from build123d import *

# Parameters (mm, degrees)
DODANIE_WYCI_GNI_CIE1_DEPTH = 20
SZKIC2_W                    = 20
SZKIC2_H                    = 40
DODANIE_WYCI_GNI_CIE2_DEPTH = 20
WYTNIJ_WYCI_GNI_CIE1_DEPTH  = 20
ZAOKR_GLENIE1_R             = 10
ZAOKR_GLENIE2_R             = 10


with BuildPart() as part:
    # Szkic1 → Dodanie-wyciągnięcie1 (new body)
    with BuildSketch(Plane.XY):
        with BuildLine():
            Line((0, 0), (40, 0))
            Line((40, 0), (40, 20))
            ThreePointArc((40, 20), (34.142135624, 34.142135624), (20, 40))
            Line((20, 40), (0, 40))
            Line((0, 40), (0, 0))
        make_face()
    extrude(amount=DODANIE_WYCI_GNI_CIE1_DEPTH)

    # Szkic2 → Dodanie-wyciągnięcie2 (add)
    with BuildSketch(Plane.XY.offset(20)):
        with Locations((10, 20)):
            Rectangle(SZKIC2_W, SZKIC2_H)
    extrude(amount=DODANIE_WYCI_GNI_CIE2_DEPTH)

    # Szkic3 → Wytnij-wyciągnięcie1 (cut)
    with BuildSketch(Plane(origin=(20, 0, 0), x_dir=(0, 0, -1), z_dir=(1, 0, 0))):
        Polygon((-40, 20), (-30, 20), (-20, 20), (-20, 40), (-40, 40), align=None)
    extrude(amount=-WYTNIJ_WYCI_GNI_CIE1_DEPTH, mode=Mode.SUBTRACT)

    # Zaokrąglenie1
    zaokr_glenie1_edges = [part.edges().sort_by_distance(p)[0] for p in [
        (10, 20, 20),
    ]]
    fillet(zaokr_glenie1_edges, radius=ZAOKR_GLENIE1_R)

    # Zaokrąglenie2
    zaokr_glenie2_edges = [part.edges().sort_by_distance(p)[0] for p in [
        (10, 20, 40),
    ]]
    fillet(zaokr_glenie2_edges, radius=ZAOKR_GLENIE2_R - 0.0001)  # a hair under: the kernel refuses the full size


solid = part.part
Read the model definition and answer for the solid it produces. Units are mm, in the model's axes. A direction names the side the tool comes from. Round coordinates to 2 decimals unless told otherwise and drop trailing zeros. Write each loop counter-clockwise with the first axis right and the second up, starting at its lowest first coordinate (ties: lowest second). Pieces come first, ordered by that corner, then holes. Notation, with made-up numbers: (3.25, -3) - (58.25, -3) arc R23 cw to (58.25, 21) - close; hole circle Ø2 at (83, 16.5). An arc over 180 degrees is marked (long way). One line per question, with ' | ' between items. Start each with the question number.
1. Section C-C (z = 19) is taken. Determine the outline of the cut face in (x, y), and give its area (3 significant figures).
2. Section D-D (y = 32) is taken. Determine the outline of the cut face in (x, z).
3. Section B-B (y = 3) is taken. Determine the outline of the cut face in (x, z), and give its area (3 significant figures).
4. Find the intervals of material crossed by probe 1 along X at (y, z) = (12.5, 24); probe 2 along Z at (x, y) = (14, 10.5), in increasing order. Write a range as [from, to].
5. For faces 1 (the face through (20, 11, 30)), 2 (the face through (15, 0, 15)), 3 (the face through (25, 20, 20)), determine the directions among +Z, -Z, +X, -X, +Y, -Y from which every point of the face is accessible in a straight line to the end or side of a thin tool.
6. Each of these flat-tipped pins is pushed along its axis until it touches: pin 1 (10 mm diameter, centred on x = 13.5, y = 21.5, fed in from -Z); pin 2 (1 mm diameter, centred on x = 12.5, y = 32, fed in from +Z); pin 3 (6 mm diameter, centred on y = 33, z = 8.5, fed in from +X); pin 4 (6 mm diameter, centred on y = 23.5, z = 17.5, fed in from +X). Where does it stop, or does it pass through?
Filled in:
1) outline: (0, 0) - (40, 0) - (40, 20) arc R20 ccw to (20, 40) - (0, 40) - close | area: 1,510 mm²
2) outline: (0, 0) - (36, 0) - (36, 20) - (0, 20) - close
3) outline: (0, 0) - (40, 0) - (40, 20) - (20, 20) - (20, 40) - (0, 40) - close | area: 1,200 mm²
4) probe 1: [0, 20] | probe 2: [0, 39.99]
5) face 1: +Z, +X, +Y, -Y | face 2: +Z, -Z, +X, -X, -Y | face 3: +Z, +X, +Y
6) pin 1: z = 0 | pin 2: z = 20 | pin 3: x = 37.32 | pin 4: x = 39.99
